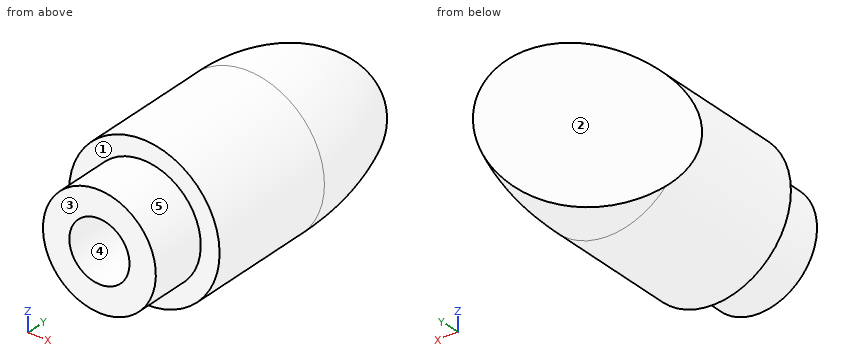
from build123d import *

# Parameters (mm, degrees)
SKETCH1_R               = 4
CUT_EXTRUDE1_START      = -3
SKETCH3_R               = 4
SKETCH3_R_2             = 3
CUT_EXTRUDE1_DEPTH      = 3
SKETCH4_R               = 4
SKETCH4_R_2             = 3
CUT_EXTRUDE2_DEPTH      = 3
SKETCH5_R               = 1.6
CUT_EXTRUDE3_DEPTH      = 10
SKETCH6_R               = 1.6
CUT_EXTRUDE4_DEPTH      = 10
CUT_EXTRUDE5_DEPTH      = 32.496031585
CUT_EXTRUDE5_DEPTH_BACK = 32.496031585
SKETCH14_R              = 1.5
BOSS_EXTRUDE4_DEPTH     = 10
SKETCH15_W              = 82.307095059
SKETCH15_H              = 58.72366942
CUT_EXTRUDE6_DEPTH      = 23.510122874


with BuildPart() as part:
    # Sweep1: sweep along a path in Sketch2
    with BuildLine(Plane.XY) as sweep1_path:
        Line((0, 0), (0, 10))
        ThreePointArc((0, 10), (-2.928932188, 17.071067812), (-10, 20))
        Line((-10, 20), (-20, 20))
    # Sketch1 → Sweep1 (sweep)
    with BuildSketch(Plane(origin=(0, 0, 0), x_dir=(1, 0, 0), z_dir=(0, 1, 0))):
        Circle(SKETCH1_R)
    sweep(path=sweep1_path.line)

    # Sketch3 → Cut-Extrude1 (cut)
    with BuildSketch(Plane.XZ.offset(CUT_EXTRUDE1_START)):
        Circle(SKETCH3_R)
        with Locations(Location((0, 0, 0), (0, 0, 270))):
            Circle(SKETCH3_R_2, mode=Mode.SUBTRACT)
    extrude(amount=CUT_EXTRUDE1_DEPTH, mode=Mode.SUBTRACT)

    # Sketch4 → Cut-Extrude2 (cut)
    with BuildSketch(Plane.ZY.offset(20)):
        with Locations(Location((0, 20, 0), (0, 0, 270))):
            Circle(SKETCH4_R)
        with Locations(Location((0, 20, 0), (0, 0, 270))):
            Circle(SKETCH4_R_2, mode=Mode.SUBTRACT)
    extrude(amount=-CUT_EXTRUDE2_DEPTH, mode=Mode.SUBTRACT)

    # Sketch5 → Cut-Extrude3 (cut)
    with BuildSketch(Plane.XZ):
        with Locations(Location((0, 0, 0), (0, 0, 270))):
            Circle(SKETCH5_R)
    extrude(amount=-CUT_EXTRUDE3_DEPTH, mode=Mode.SUBTRACT)

    # Sketch6 → Cut-Extrude4 (cut)
    with BuildSketch(Plane.ZY.offset(20)):
        with Locations(Location((0, 20, 0), (0, 0, 270))):
            Circle(SKETCH6_R)
    extrude(amount=-CUT_EXTRUDE4_DEPTH, mode=Mode.SUBTRACT)

    # Sketch11 → Cut-Extrude5 (cut, two sides: drawn at the far end of the back side and taken through both)
    with BuildSketch(Plane.XY.offset(-CUT_EXTRUDE5_DEPTH_BACK)):
        Polygon((-15.076530842, 11.99453697), (5.142966103, 32.214033915), (12.214033915, 25.142966103), (-8.00546303, 4.923469158), align=None)
    extrude(amount=CUT_EXTRUDE5_DEPTH + CUT_EXTRUDE5_DEPTH_BACK, mode=Mode.SUBTRACT)


with BuildPart() as cut_extrude5_piece_1:
    # of the separate pieces the step leaves, piece 1, a body of its own (cut_extrude5_pieces)
    add(part.part.solids().sort_by_distance((4, 3, 0))[0])



with BuildPart() as cut_extrude5_piece_2:
    # of the separate pieces the step leaves, piece 2, a body of its own (cut_extrude5_pieces)
    add(part.part.solids().sort_by_distance((-10, 17.071067812, -2.724216628))[0])


with BuildPart() as cut_extrude5_piece_1_1:
    add(cut_extrude5_piece_1.part)

    add(cut_extrude5_piece_2.part)  # Boss-Extrude4 merges Cut-Extrude5 piece 2
    # Sketch14 → Boss-Extrude4 (add)
    with BuildSketch(Plane(origin=(-6.464466094, 6.464466094, 0), x_dir=(0, 0, 1), z_dir=(-0.7071067811865517, 0.7071067811865434, 0))):
        with Locations(Location((0, 9.142135624, 0), (0, 0, 270))):
            Circle(SKETCH14_R)
    extrude(amount=BOSS_EXTRUDE4_DEPTH)

    # Sketch15 → Cut-Extrude6 (cut, through all)
    with BuildSketch(Plane(origin=(-6.464466094, 6.464466094, 0), x_dir=(0, 0, 1), z_dir=(-0.7071067811865517, 0.7071067811865434, 0))):
        with Locations((3.361016584, 6.067930336)):
            Rectangle(SKETCH15_W, SKETCH15_H)
    extrude(amount=CUT_EXTRUDE6_DEPTH, mode=Mode.SUBTRACT)


solid = cut_extrude5_piece_1_1.part
For this review, take the finished solid that the model builds, in its own axes (mm). Face numbers are marked on the shaded views. A direction names the side the tool comes from. Round coordinates to 2 decimals unless told otherwise and drop trailing zeros. Order: outer loops, then holes, each group sorted by start corner. A loop starts at its lowest first (then second) coordinate and runs counter-clockwise, first axis right, second up. Notation, with made-up numbers: M 78.25,-17.75 L 89.25,-17.75 A17 ccw 89.25,2.25 Z; hole C 17,54 d10. An arc over 180 degrees is marked long. Use a Markdown table: item, result. Add a question column.
Item 1: Tool access review of the marked faces 1 and 2: name each direction out of +Z, -Z, +X, -X, +Y, -Y from which nothing blocks a thin tool from reaching the whole face with its end or side.
Item 2: To check wall thickness, follow line 1 along X through (y, z) = (2, 0); line 2 along X through (y, z) = (4.25, 0); line 3 along Z through (x, y) = (1, 8.5). State the ranges of each line that lie inside material, in increasing order.
Item 3: Insertion check: pin 1 (2 mm diameter, centred on y = 5.5, z = -3, fed in from -X); pin 2 (1 mm diameter, centred on x = 3, z = 1, fed in from +Y); pin 3 (1 mm diameter, centred on y = 11, z = -3, fed in from +X). Each pin has a flat end and moves straight along its axis. Give the tip position at first contact, or say it passes through.
Item 4: Add section D-D, the plane y = 9.5. Give the boundary of the cut face in (x, z), then the cut area to 3 significant figures.
Item 5: Add section A-A, the plane z = 0. Give the boundary of the cut face in (x, y).
Item 6: Mouldability with a two-part tool opening along Z and no side actions: class the marked faces 3, 4 and 5 as released by +Z, released by -Z, zero draft, split by the parting line, or undercut.
Item 7: Add section C-C, the plane z = -3.25. Give the boundary of the cut face in (x, y), then the cut area to 3 significant figures.
Item 8: Add section B-B, the plane y = 3.25. Give the boundary of the cut face in (x, z).
Geometry results:
| question | item | result |
|---|---|---|
| 1 | face 1 | -Y |
| 1 | face 2 | +Z, -Z, -X, +Y |
| 2 | line 1 | x = -3 to -1.6, 1.6 to 3 |
| 2 | line 2 | x = -4 to -1.6, 1.6 to 4 |
| 2 | line 3 | z = -3.87 to -1.25, 1.25 to 3.87 |
| 3 | pin 1 | stops at x = -3.46 |
| 3 | pin 2 | stops at y = 15.68 |
| 3 | pin 3 | stops at x = 3.09 |
| 4 | outline | M -3.43,-2.06 A4 ccw long -3.43,2.06 Z; hole C 0,0 d3.2 |
| 4 | area | 40.6 mm² |
| 5 | outline | M -4,3 L -3,3 L -3,0 L -1.6,0 L -1.6,10 L 1.6,10 L 1.6,0 L 3,0 L 3,3 L 4,3 L 4,10 A14 ccw 2.78,15.71 L -4,8.93 Z |
| 6 | face 3 | zero draft |
| 6 | face 4 | undercut |
| 6 | face 5 | split by the parting line |
| 7 | outline | M -2.35,10.58 A7.67 cw -2.33,10 L -2.33,3 L 2.33,3 L 2.33,10 A12.33 ccw 1.51,14.44 Z |
| 7 | area | 44.8 mm² |
| 8 | outline | C 0,0 d8; hole C 0,0 d3.2 |
